Verification items for the finished model (mm, model axes). Coordinates: 2 decimals unless noted, no trailing zeros. Order: outer loops, then holes, each group sorted by start corner. A loop starts at its lowest first (then second) coordinate and runs counter-clockwise, first axis right, second up. Notation, with made-up numbers: M 28,88 L 40,88 A17 cw 40,99 Z; hole C 73,-40 d7. An arc over 180 degrees is marked long. Write item = value, one per line.
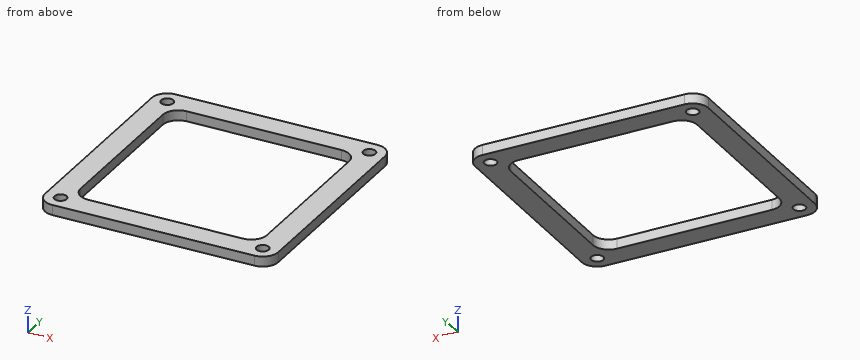
```python
from build123d import *

# Parameters (mm, degrees)
MODEL_R         = 1.575
EXTRUDE_1_DEPTH = 2.6


with BuildPart() as part:
    # Model → 凸台-拉伸1 (new body)
    with BuildSketch(Plane.XY):
        with BuildLine():
            Line((2267.087112804, 1815.358905475), (2267.087112804, 1763.358905475))
            ThreePointArc((2267.087112804, 1763.358905475), (2268.25868568, 1760.53047835), (2271.087112804, 1759.358905475))
            Line((2271.087112804, 1759.358905475), (2323.087112804, 1759.358905475))
            ThreePointArc((2323.087112804, 1759.358905475), (2325.915539929, 1760.53047835), (2327.087112804, 1763.358905475))
            Line((2327.087112804, 1763.358905475), (2327.087112804, 1815.358905475))
            ThreePointArc((2327.087112804, 1815.358905475), (2325.915539929, 1818.187332599), (2323.087112804, 1819.358905475))
            Line((2323.087112804, 1819.358905475), (2271.087112804, 1819.358905475))
            ThreePointArc((2271.087112804, 1819.358905475), (2268.25868568, 1818.187332599), (2267.087112804, 1815.358905475))
        make_face()
        with Locations((2271.087112804, 1763.358905475)):
            Circle(MODEL_R, mode=Mode.SUBTRACT)
        with Locations((2323.087112804, 1763.358905475)):
            Circle(MODEL_R, mode=Mode.SUBTRACT)
        with Locations((2271.087112804, 1815.358905475)):
            Circle(MODEL_R, mode=Mode.SUBTRACT)
        with Locations((2323.087112804, 1815.358905475)):
            Circle(MODEL_R, mode=Mode.SUBTRACT)
        with BuildLine():
            Line((2295.483483019, 1813.357611428), (2317.000502455, 1813.357611428))
            ThreePointArc((2317.000502455, 1813.357611428), (2319.828929579, 1812.186038553), (2321.000502455, 1809.357611428))
            Line((2321.000502455, 1809.357611428), (2321.000502455, 1769.362445027))
            ThreePointArc((2321.000502455, 1769.362445027), (2319.828929579, 1766.534017903), (2317.000502455, 1765.362445027))
            Line((2317.000502455, 1765.362445027), (2277.087112804, 1765.362445027))
            ThreePointArc((2277.087112804, 1765.362445027), (2274.25868568, 1766.534017903), (2273.087112804, 1769.362445027))
            Line((2273.087112804, 1769.362445027), (2273.087112804, 1809.357611428))
            ThreePointArc((2273.087112804, 1809.357611428), (2274.25868568, 1812.186038553), (2277.087112804, 1813.357611428))
            Line((2277.087112804, 1813.357611428), (2295.483483019, 1813.357611428))
        make_face(mode=Mode.SUBTRACT)
    extrude(amount=EXTRUDE_1_DEPTH)


solid = part.part
```
Item 1: Sectioned sample at C-C, the plane z = 1.25. Give the number of separate pieces and of enclosed holes in the cut face, then the cut area to 3 significant figures.
Report:
separate_pieces = 1
enclosed_holes = 5
area = 1,270 mm^2
Item 2: Sectioned sample at B-B, the plane y = 1800. Enter the section's corners in (x, z), then the cut area to 3 significant figures.
Report:
outline = M 2267.09,0 L 2273.09,0 L 2273.09,2.6 L 2267.09,2.6 Z; M 2321,0 L 2327.09,0 L 2327.09,2.6 L 2321,2.6 Z
area = 31.4 mm^2
Item 3: Gauge pin test, flat end, axial feed: pin 1 (2.5 mm diameter, centred on x = 2271.09, y = 1815.36, fed in from -Z). Record the tip position at first contact, or that the pin passes through.
Report:
pin_1 = through
Item 4: Sectioned sample at A-A, the plane x = 2286.5. Enter the section's corners in (y, z), then the cut area to 3 significant figures.
Report:
outline = M 1759.36,0 L 1765.36,0 L 1765.36,2.6 L 1759.36,2.6 Z; M 1813.36,0 L 1819.36,0 L 1819.36,2.6 L 1813.36,2.6 Z
area = 31.2 mm^2
Item 5: Scan lines: L1, parallel to X at y = 1776, z = 1.6; L2, parallel to Y at x = 2282.5, z = 0.6; L3, parallel to Y at x = 2270.5, z = 0.45. Record each from-to range of solid material in increasing order. Write a range as from..to.
Report:
L1 = 2267.09..2273.09, 2321..2327.09
L2 = 1759.36..1765.36, 1813.36..1819.36
L3 = 1759.4..1761.9, 1764.82..1813.9, 1816.82..1819.32
